```python
from build123d import *

# Parameters (mm, degrees)
SKETCH_W              = 399.99
SKETCH_H              = 399.99
PAD_DEPTH             = 15
SKETCH001_R           = 6
POCKET_DEPTH          = 1146.741253
SKETCH002_R           = 2
POCKET001_DEPTH       = 1146.741253
POLARPATTERN_COUNT    = 16
POLARPATTERN001_COUNT = 2


with BuildPart() as part:
    # Sketch → Pad (new body)
    with BuildSketch(Plane.XY):
        Rectangle(SKETCH_W, SKETCH_H)
    extrude(amount=PAD_DEPTH)

    # Sketch001 (on Face6 of Pad) → Pocket (cut, through all)
    with BuildSketch(Plane.XY.offset(15)):
        with Locations((0, 50)):
            Circle(SKETCH001_R)
    pocket = extrude(amount=-POCKET_DEPTH, mode=Mode.SUBTRACT)

    # Sketch002 (on Face5 of Pocket) → Pocket001 (cut, through all)
    with BuildSketch(Plane.XY.offset(15)):
        with Locations((0, 177)):
            Circle(SKETCH002_R)
    pocket001 = extrude(amount=-POCKET001_DEPTH, mode=Mode.SUBTRACT)

    # PolarPattern: Pocket001 ×16 about axis
    polarpattern_axis = Axis((0, 0, 15), (0, 0, 1))
    for i in range(1, POLARPATTERN_COUNT):
        add(pocket001.rotate(polarpattern_axis, i * 360 / POLARPATTERN_COUNT), mode=Mode.SUBTRACT)

    # PolarPattern001: Pocket ×2 about axis
    polarpattern001_axis = Axis((0, 0, 15), (0, 0, 1))
    for i in range(1, POLARPATTERN001_COUNT):
        add(pocket.rotate(polarpattern001_axis, i * 360 / POLARPATTERN001_COUNT), mode=Mode.SUBTRACT)


solid = part.part
```
Build history of the part. All positions in model axes, mm. Round coordinates to 2 decimals unless told otherwise and drop trailing zeros. Write each loop counter-clockwise with the first axis right and the second up, starting at its lowest first coordinate (ties: lowest second). Pieces come first, ordered by that corner, then holes.
1) Mould opens along Y. For faces 1 (the flat face through (199.995, -3, 7)), 2 (the flat face through (-3, 199.995, 7)), 3 (the cylindrical face through (1.301, -44.143, 7.605)) say: +Y half, -Y half, draft (parallel to the pull), parting line (faces both ways), or undercut.
2) Drill centre lines: probe 1 along Y at (x, z) = (0, 8.75) (3 decimals); probe 2 along X at (y, z) = (0, 8) (3 decimals); probe 3 along X at (y, z) = (-51, 2.5) (3 decimals). Where is each one in solid material? Low to high.
3) Band-saw the part on A-A, the plane y = 50. List the corners of the cut face in (x, z) (3 decimals), and give its area (3 significant figures).
Ans:
1. face 1: draft
1. face 2: +Y half
1. face 3: undercut
2. probe 1: y = -199.995 to -179, -175 to -56, -44 to 44, 56 to 175, 179 to 199.995
2. probe 2: x = -199.995 to -179, -175 to 175, 179 to 199.995
2. probe 3: x = -199.995 to -5.916, 5.916 to 199.995
3. outline: (-199.995, 0) - (-6, 0) - (-6, 15) - (-199.995, 15) - close; (6, 0) - (199.995, 0) - (199.995, 15) - (6, 15) - close
3. area: 5,820 mm2
